```python
from build123d import *

# Parameters (mm, degrees)
BOSS_EXTRUDE1_DEPTH                                 = 9.525
CSK_FOR_1_4_FLAT_HEAD_MACHINE_SCREW_100_D           = 6.7564
CSK_FOR_1_4_FLAT_HEAD_MACHINE_SCREW_100_CSINK_D     = 17.6447958
CSK_FOR_1_4_FLAT_HEAD_MACHINE_SCREW_100_CSINK_ANGLE = 100
LPATTERN1_COUNT                                     = 2
LPATTERN1_PITCH                                     = 491.2
LPATTERN1_COUNT_DIR2                                = 5
LPATTERN1_PITCH_DIR2                                = 287.65
LPATTERN2_COUNT                                     = 3
LPATTERN2_PITCH                                     = 163.733333333
LPATTERN2_COUNT_DIR2                                = 2
LPATTERN2_PITCH_DIR2                                = 76.2
FILLET1_R                                           = 3.175


with BuildPart() as part:
    # Sketch1 → Boss-Extrude1 (new body)
    with BuildSketch(Plane(origin=(0, 0, 0), x_dir=(1, 0, 0), z_dir=(0, 1, 0))):
        Polygon((-258.3, 0), (-207.5, 0), (-207.5, 1074.4), (207.5, 1074.4), (207.5, 0), (258.3, 0), (258.3, 1113.914856628), (230.3, 1117.85), (-61.7, 1117.85), (-61.7, 1132.55), (271.3, 1132.55), (271.3, 1176), (-258.3, 1176), align=None)
    extrude(amount=BOSS_EXTRUDE1_DEPTH)

    # CSK for 1_4 Flat Head Machine Screw _100 (through all)
    with Locations(Plane.XZ):
        with Locations((-245.6, -1163.3)):
            csk_for_1_4_flat_head_machine_screw_100 = CounterSinkHole(CSK_FOR_1_4_FLAT_HEAD_MACHINE_SCREW_100_D / 2, CSK_FOR_1_4_FLAT_HEAD_MACHINE_SCREW_100_CSINK_D / 2, counter_sink_angle=CSK_FOR_1_4_FLAT_HEAD_MACHINE_SCREW_100_CSINK_ANGLE)

    # LPattern1: CSK for 1_4 Flat Head Machine Screw _100 2 × 5
    with Locations(*[(i * LPATTERN1_PITCH, 0, j * LPATTERN1_PITCH_DIR2) for i in range(LPATTERN1_COUNT) for j in range(LPATTERN1_COUNT_DIR2) if (i, j) != (0, 0)]):
        add(csk_for_1_4_flat_head_machine_screw_100, mode=Mode.SUBTRACT)

    # LPattern2: CSK for 1_4 Flat Head Machine Screw _100 3 × 2, 1 skipped
    with Locations(*[(i * LPATTERN2_PITCH, 0, j * LPATTERN2_PITCH_DIR2) for i in range(LPATTERN2_COUNT) for j in range(LPATTERN2_COUNT_DIR2) if (i, j) not in ((0, 0), (0, 1))]):
        add(csk_for_1_4_flat_head_machine_screw_100, mode=Mode.SUBTRACT)

    # Fillet1
    fillet1_edges = [part.edges().sort_by_distance(p)[0] for p in [
        (-207.5, 4.7625, 0),
        (-258.3, 4.7625, 0),
        (271.3, 4.7625, -1176),
        (271.3, 4.7625, -1132.55),
        (-61.7, 4.7625, -1132.55),
        (-61.7, 4.7625, -1117.85),
        (258.3, 4.7625, -1113.914856628),
        (258.3, 4.7625, 0),
        (207.5, 4.7625, 0),
        (207.5, 4.7625, -1074.4),
        (-207.5, 4.7625, -1074.4),
    ]]
    fillet(fillet1_edges, radius=FILLET1_R)


solid = part.part
```
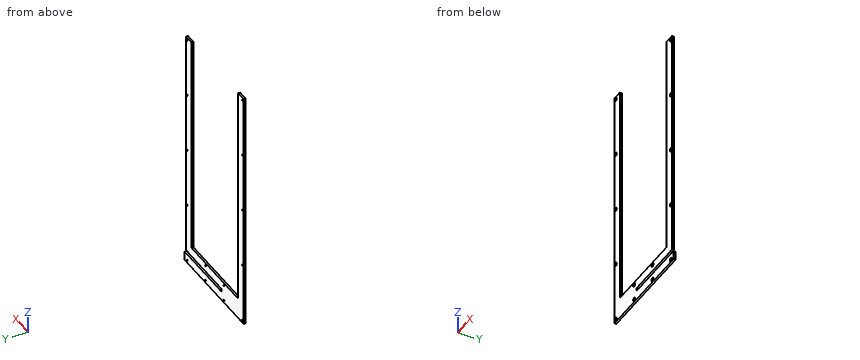
Geometry check sheet. Reference: the model listing, model coordinates, mm. Round coordinates to 2 decimals unless told otherwise and drop trailing zeros. Order: outer loops, then holes, each group sorted by start corner. A loop starts at its lowest first (then second) coordinate and runs counter-clockwise, first axis right, second up. Notation, with made-up numbers: (2, 46) -> (59, 46) arc R36 cw to (59, 82) -> close; hole circle Ø6 at (48.25, 10). An arc over 180 degrees is marked (long way). Return JSON: item names as keys, results as strings. Group by question number.
Q1. Section check A-A, the plane x = -22. Record the boundary of the cut face in (y, z) (3 decimals), plus the area to 3 significant figures.
Q2. Section check B-B, the plane z = -811. Record the boundary of the cut face in (x, y) (3 decimals), plus the area to 3 significant figures.
Q3. Material ranges on probe 1 along Z at (x, y) = (-245.6, 8.5); probe 2 along X at (y, z) = (8.4, -1163.3); probe 3 along X at (y, z) = (6.9, -300.35), recorded low to high. Write a range as from..to.
Q4. Section check C-C, the plane y = 6.75. Count the separate pieces of the cut face and the enclosed holes in it, plus the area to 3 significant figures.
Q5. Section check D-D, the plane x = -169. Record the boundary of the cut face in (y, z) (3 decimals), plus the area to 3 significant figures.
Q6. Gauge pin test, flat ends, axial feed: pin 1 (3 mm diameter, centred on x = -39, y = 3.5, fed in from +Z); pin 2 (9 mm diameter, centred on x = 245.6, z = -588, fed in from -Y); pin 3 (11 mm diameter, centred on x = -245.6, z = -875.65, fed in from -Y). Record the tip position at first contact, or that the pin passes through.
Numbers:
{
 "1": {"outline": "(0, -1176) -> (9.525, -1176) -> (9.525, -1132.55) -> (0, -1132.55) -> close; (0, -1117.85) -> (9.525, -1117.85) -> (9.525, -1074.4) -> (0, -1074.4) -> close", "area": "828 mm^2"},
 "2": {"outline": "(-258.3, 0) -> (-207.5, 0) -> (-207.5, 9.525) -> (-258.3, 9.525) -> close; (207.5, 0) -> (258.3, 0) -> (258.3, 9.525) -> (207.5, 9.525) -> close", "area": "968 mm^2"},
 "3": {"probe 1": "-1176..-1166.68, -1159.92..-879.03, -872.27..-591.38, -584.62..-303.73, -296.97..-16.08, -9.32..0", "probe 2": "-258.3..-248.98, -242.22..-85.24, -78.49..78.49, 85.24..242.22, 248.98..271.3", "probe 3": "-258.3..-248.98, -242.22..-207.5, 207.5..242.22, 248.98..258.3"},
 "4": {"separate pieces": "1", "enclosed holes": "14", "area": "157,000 mm^2"},
 "5": {"outline": "(0, -1176) -> (9.525, -1176) -> (9.525, -1074.4) -> (0, -1074.4) -> close", "area": "968 mm^2"},
 "6": {"pin 1": "z = -1074.4", "pin 2": "y = 3.63", "pin 3": "y = 2.79"}
}
